from build123d import *

# Parameters (mm, degrees)
F0_W     = 58
F0_H     = 22
F1_DEPTH = 10
F2_R     = 2
F3_DEPTH = 25
F4_R     = 1.5
F5_DEPTH = 500
F6_W     = 38
F6_H     = 10
F7_DEPTH = 10
F8_R     = 2
F9_DEPTH = 25


with BuildPart() as f1:
    # F0 (on Top) → F1 (new body)
    with BuildSketch(Plane.XY):
        Rectangle(F0_W, F0_H)
    extrude(amount=F1_DEPTH)

    # F2 (on face) → F3 (cut)
    with BuildSketch(Plane.XY.offset(10)):
        with Locations((-19.5, -4)):
            Circle(F2_R)
        with Locations((19.5, -4)):
            Circle(F2_R)
    extrude(amount=-F3_DEPTH, mode=Mode.SUBTRACT)

    # F4 (on face) → F5 (cut)
    with BuildSketch(Plane.YZ.offset(29)):
        with Locations((7, 2)):
            Circle(F4_R)
    extrude(amount=-F5_DEPTH, mode=Mode.SUBTRACT)

    # F6 (on face) → F7 (join)
    with BuildSketch(Plane(origin=(0, 11, 0), x_dir=(-1, 0, 0), z_dir=(0, 1, 0))):
        with Locations((0, 5)):
            Rectangle(F6_W, F6_H)
    extrude(amount=F7_DEPTH)

    # F8 (on face) → F9 (cut)
    with BuildSketch(Plane.XY.offset(10)):
        with Locations((12, 17)):
            Circle(F8_R)
        with Locations((-12, 16)):
            Circle(F8_R)
    extrude(amount=-F9_DEPTH, mode=Mode.SUBTRACT)


solid = f1.part
Read the model definition and answer for the solid it produces. Units are mm, in the model's axes. A direction names the side the tool comes from. Give positions to 0.01 mm unless a question says otherwise; leave off trailing zeros. Write each loop counter-clockwise with the first axis right and the second up, starting at its lowest first coordinate (ties: lowest second). Pieces come first, ordered by that corner, then holes. Notation, with made-up numbers: (24, 10) - (35, 10) arc R15 cw to (35, 26) - close; hole circle Ø1 at (89, -3.5). An arc over 180 degrees is marked (long way). Use CSV: the item, a comma, the result in double quotes. Start each with the question number.
(1) Determine the mould class of faces 1 (the flat face through (0, 5, 0)), 2 (the flat face through (-29, 0, 5)), 3 (the cylindrical face through (0.4, 5.8, 1.1)) for opening direction Z: +Z half, -Z half, draft (parallel to the pull), parting line (faces both ways), or undercut.
(2) Find section B-B (z = 2.75). Give the vertices of the cut face in (x, y).
(3) Find section D-D (x = 22.5). Give the vertices of the cut face in (y, z).
(4) Given P1, Ø2, axis at x = 10, y = 15, coming from the -Z side; P2, Ø3, axis at y = 17.5, z = 5.5, coming from the +X side; P3, Ø3, axis at x = -25.5, z = 6.5, coming from the +Y side; P4, Ø2.5, axis at x = 19.5, y = -4, coming from the -Z side, each flat-ended and moving along its own axis, determine where each tip first touches the part or whether it passes through.
(5) Consider line 1 along Y through (x, z) = (-12, 3.75); line 2 along Y through (x, z) = (12, 7.75); line 3 along Y through (x, z) = (-12, 2.5). Determine where each line is inside the solid, lowest interval first.
(6) Find section C-C (y = 7). Give the vertices of the cut face in (x, z), plus the area to 3 significant figures.
(7) For faces 4 (the flat face through (24, 11, 5)), 5 (the flat face through (-24, 11, 5)), 6 (the cylindrical face through (12, 19, 5)), determine the directions among +Z, -Z, +X, -X, +Y, -Y from which every point of the face is accessible in a straight line to the end or side of a thin tool.
(8) Find section A-A (x = 12). Give the vertices of the cut face in (y, z).
Findings below:
1,face 1,"-Z half"
1,face 2,"draft"
1,face 3,"undercut"
2,outline,"(-29, -11) - (29, -11) - (29, 5.7) - (-29, 5.7) - close; (-29, 8.3) - (29, 8.3) - (29, 11) - (19, 11) - (19, 21) - (-19, 21) - (-19, 11) - (-29, 11) - close; hole circle Ø4 at (-19.5, -4); hole circle Ø4 at (-12, 16); hole circle Ø4 at (12, 17); hole circle Ø4 at (19.5, -4)"
3,outline,"(-11, 0) - (11, 0) - (11, 10) - (-11, 10) - close; hole circle Ø3 at (7, 2)"
4,P1,"z = 0"
4,P2,"x = 19"
4,P3,"y = 11"
4,P4,"through"
5,line 1,"-11 to 14, 18 to 21"
5,line 2,"-11 to 15, 19 to 21"
5,line 3,"-11 to 5.59, 8.41 to 14, 18 to 21"
6,outline,"(-29, 0) - (29, 0) - (29, 0.5) - (-29, 0.5) - close; (-29, 3.5) - (29, 3.5) - (29, 10) - (-29, 10) - close"
6,area,"406 mm2"
7,face 4,"+Z, -Z, +X, +Y"
7,face 5,"+Z, -Z, -X, +Y"
7,face 6,"+Z, -Z"
8,outline,"(-11, 0) - (15, 0) - (15, 10) - (-11, 10) - close; (19, 0) - (21, 0) - (21, 10) - (19, 10) - close; hole circle Ø3 at (7, 2)"
